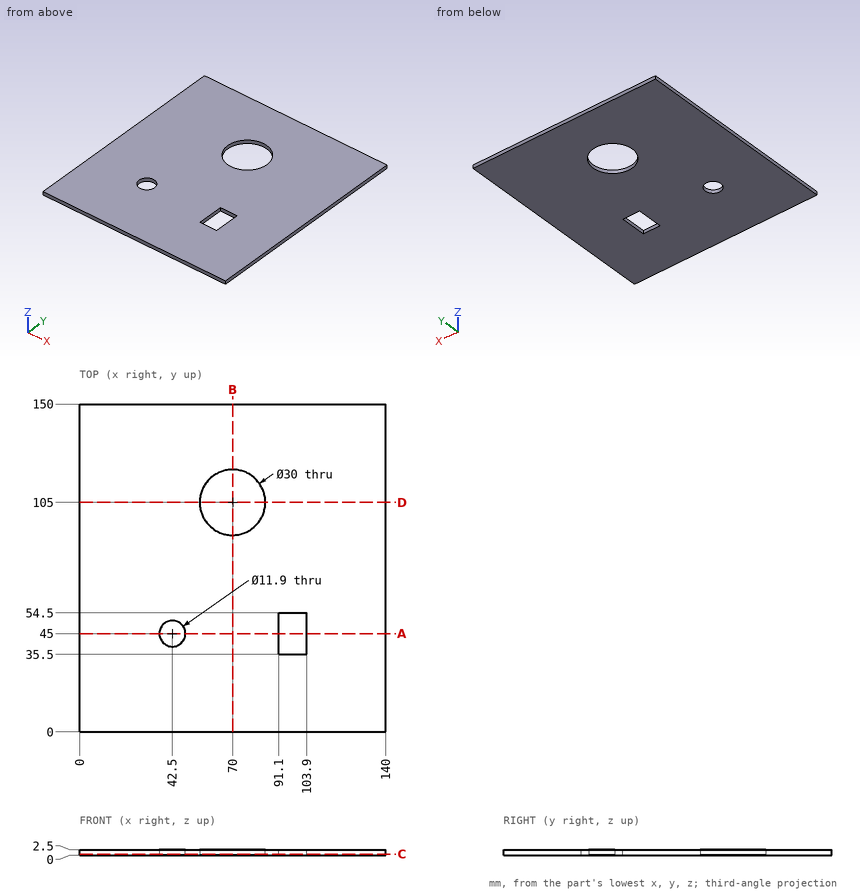
Drawing for the job (mm, zero at the part's lowest x, y, z). Round coordinates to 2 decimals unless told otherwise and drop trailing zeros. Order: outer loops, then holes, each group sorted by start corner. A loop starts at its lowest first (then second) coordinate and runs counter-clockwise, first axis right, second up. Notation, with made-up numbers: M 23,-17.5 L 49,-17.5 A19 cw 49,0.5 Z; hole C -17.5,-39.5 d7. An arc over 180 degrees is marked long. Use one line per item in the form item = value.
Q1. Saw through at A-A on y = 45. Give the cut face in (x, z).
Recorded:
outline = M 0,0 L 36.55,0 L 36.55,2.5 L 0,2.5 Z; M 48.45,0 L 91.1,0 L 91.1,2.5 L 48.45,2.5 Z; M 103.9,0 L 140,0 L 140,2.5 L 103.9,2.5 Z
Q2. Probe L1, parallel to Y at x = 70, z = 1.15; L2, parallel to Y at x = 42.5, z = 1.1; L3, parallel to X at y = 106, z = 1.7. List the from-to ranges inside material, lowest first.
Recorded:
L1 = 0 to 90, 120 to 150
L2 = 0 to 39.05, 50.95 to 150
L3 = 0 to 55.03, 84.97 to 140
Q3. Saw through at B-B on x = 70. Give the cut face in (y, z).
Recorded:
outline = M 0,0 L 90,0 L 90,2.5 L 0,2.5 Z; M 120,0 L 150,0 L 150,2.5 L 120,2.5 Z
Q4. Flat gauge pin, fed straight in: P1, Ø7, axis at x = 42.5, y = 45, coming from the -Z side. Where does the tip first touch, or does it go through?
Recorded:
P1 = through
Q5. Saw through at D-D on y = 105. Give the cut face in (x, z).
Recorded:
outline = M 0,0 L 55,0 L 55,2.5 L 0,2.5 Z; M 85,0 L 140,0 L 140,2.5 L 85,2.5 Z
Q6. Saw through at C-C on z = 0.6. Give the cut face in (x, y).
Recorded:
outline = M 0,0 L 140,0 L 140,150 L 0,150 Z; hole C 42.5,45 d11.9; hole C 70,105 d30; hole M 91.1,35.5 L 103.9,35.5 L 103.9,54.5 L 91.1,54.5 Z
